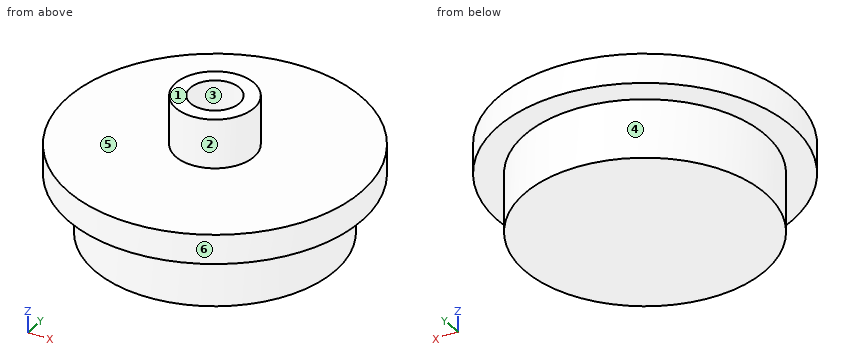
Autodesk Fusion 360 part; units mm, degrees
sketch "Sketch1" plane through (0, 0, 0) normal (0, 0, 1) x (1, 0, 0)
  circle A0 centre (0, 0) radius 12.3
  circle A1 centre (0, 0) radius 2.5
  circle A2 centre (0, 0) radius 4
  circle A3 centre (0, 0) radius 15
  dimension "d1" = 24.6
  dimension "led_diam" = 5
  dimension "d3" = 8
  dimension "d4" = 30
extrude "Extrude1" add sketch "Sketch1" along normal blind 6 contours A0 | A1 | A2
extrude "Extrude2" add sketch "Sketch1" along normal blind 3 from surface at 6 contours A0 | A1 | A2 | A3
extrude "Extrude4" add sketch "Sketch1" along normal blind 5 from surface at 9 contours A2
equation "d3 = led_diam + 3 mm"
equation "light_offset = diffuser_thick"
equation "d13 = diffuser_thick + support_thick"
Verification items for the finished model (mm, model axes). Face numbers are marked on the shaded views. A direction names the side the tool comes from. Coordinates: 2 decimals unless noted, no trailing zeros. Order: outer loops, then holes, each group sorted by start corner. A loop starts at its lowest first (then second) coordinate and runs counter-clockwise, first axis right, second up. Notation, with made-up numbers: M 36,-1.75 L 67,-1.75 A23 cw 67,19.25 Z; hole C 66,38.5 d5. An arc over 180 degrees is marked long. One line per item, written item: value. Start each with the question number.
Item 1: Access from +Z, -Z, +X, -X, +Y, -Y to the whole of each face (thin tool, end or side, straight path). Record for the marked faces 4, 5 and 6.
Item 2: Depth check by flat-ended pin: P1, Ø4.5, axis at x = 0, y = 0, coming from the +Z side; P2, Ø5, axis at y = -6, z = 3, coming from the -X side; P3, Ø3, axis at x = 2, z = 2.5, coming from the -Y side. Enter the tip coordinate at first touch or a pass-through.
Item 3: Sectioned sample at C-C on z = 2.5. Record the cut outline in (x, y), then the cut area to 3 significant figures.
Item 4: Sectioned sample at A-A on y = 0. Record the cut outline in (x, z), then the cut area to 3 significant figures.
Item 5: Mould release check, pull along X, two halves, no side actions. Record for the marked faces 1, 2 and 3: pulls with the +X half, pulls with the -X half, needs draft (parallel to the pull), parting line crosses it, or undercut.
Item 6: Thickness scan on probe 1 along Y at (x, z) = (0, 10.3); probe 2 along Z at (x, y) = (-7.5, -12); probe 3 along Z at (x, y) = (4, -8). Record the ranges inside material, lowest first.
Item 7: Sectioned sample at D-D on y = -8.25. Record the cut outline in (x, z), then the cut area to 3 significant figures.
Calculated:
1. face 4: -Z
1. face 5: +Z
1. face 6: +Z, -Z
2. P1: z = 9
2. P2: x = -11.79
2. P3: y = -12.29
3. outline: C 0,0 d24.6
3. area: 475 mm^2
4. outline: M -15,6 L -12.3,6 L -12.3,0 L 12.3,0 L 12.3,6 L 15,6 L 15,9 L 4,9 L 4,14 L 2.5,14 L 2.5,9 L -2.5,9 L -2.5,14 L -4,14 L -4,9 L -15,9 Z
4. area: 253 mm^2
5. face 1: needs draft
5. face 2: parting line crosses it
5. face 3: undercut
6. probe 1: -4 to -2.5, 2.5 to 4
6. probe 2: 6 to 9
6. probe 3: 0 to 9
7. outline: M -12.53,6 L -9.12,6 L -9.12,0 L 9.12,0 L 9.12,6 L 12.53,6 L 12.53,9 L -12.53,9 Z
7. area: 185 mm^2
